Can you work these out from the drawing? Everything is in mm from the part's minimum corner. A direction names the side the tool comes from. Round coordinates to 2 decimals unless told otherwise and drop trailing zeros. Loops run counter-clockwise (first coordinate to the right, second up) from the corner with the lowest first, then second, coordinate; pieces in that order, holes last. Notation, with made-up numbers: (55.5, 17.25) -> (64.5, 17.25) arc R6 cw to (64.5, 21.25) -> close; hole circle Ø7 at (21.5, 47). An arc over 180 degrees is marked (long way). One line per item, written item: value.
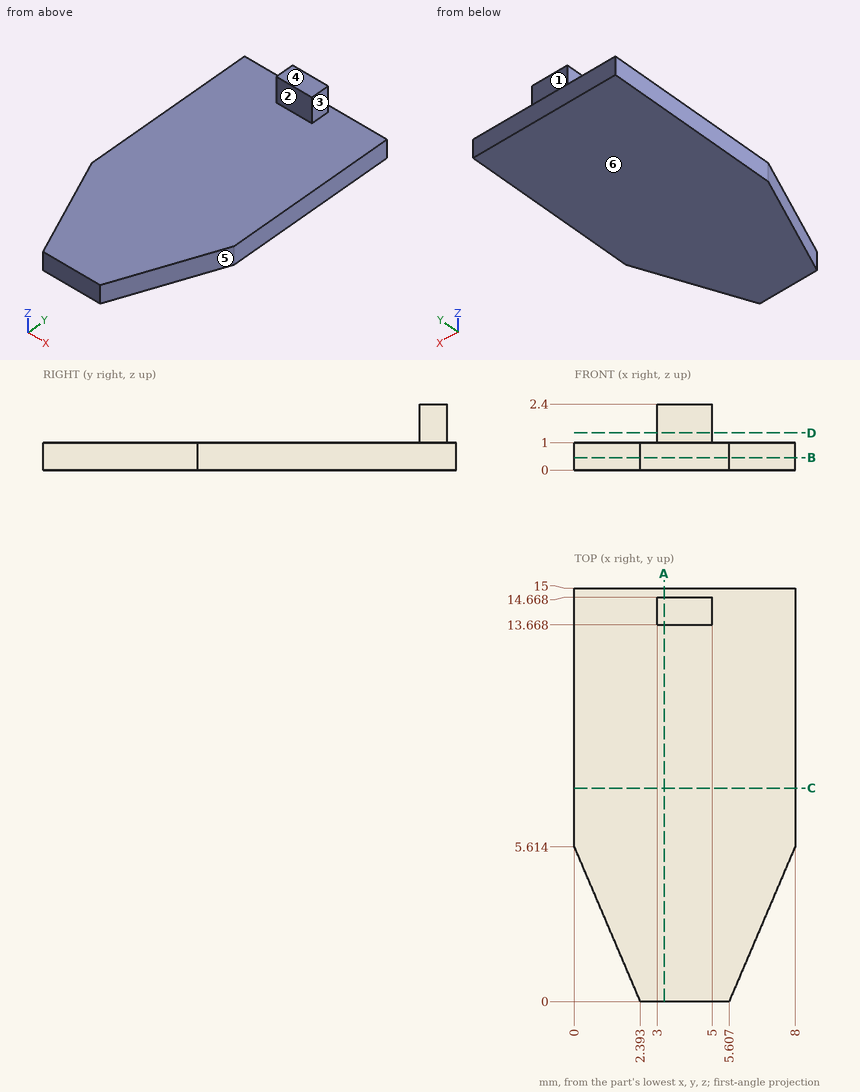
Item 1: If we section it at B-B on z = 0.45: List the corners of the cut face in (x, y) for me, plus the area to 3 significant figures.
Output:
outline: (0, 5.61) -> (2.39, 0) -> (5.61, 0) -> (8, 5.61) -> (8, 15) -> (0, 15) -> close
area: 107 mm²
Item 2: For the marked faces 1, 2 and 3, which set-ups out of +Z, -Z, +X, -X, +Y, -Y let a thin tool reach every point of the face, with its end or its side?
Output:
face 1: +Z, +X, -X, +Y
face 2: +Z, +X, -X, -Y
face 3: +Z, +X, +Y, -Y
Item 3: If we section it at C-C on y = 7.75: List the corners of the cut face in (x, z) for me.
Output:
outline: (0, 0) -> (8, 0) -> (8, 1) -> (0, 1) -> close
Item 4: Will these pins go through, and if not, where does the flat tip stop? pin 1 Ø1.1 at (x, z) = (4, 1.5) entering from +Y; pin 2 Ø1 at (x, y) = (1, 3) entering from +Z; pin 3 Ø0.7 at (x, z) = (4, 1.5) entering from -Y.
Output:
pin 1: stops at y = 15
pin 2: stops at z = 1
pin 3: stops at y = 13.67
Item 5: If we mould it in two halves opening along Z, with no side actions, what happens to the marked faces 4, 5 and 6? For each: released by +Z, released by -Z, zero draft, split by the parting line, or undercut.
Output:
face 4: released by +Z
face 5: zero draft
face 6: released by -Z
Item 6: If we section it at D-D on z = 1.35: List the corners of the cut face in (x, y) for me, plus the area to 3 significant figures.
Output:
outline: (3, 13.67) -> (5, 13.67) -> (5, 14.67) -> (3, 14.67) -> close
area: 2.00 mm²
Item 7: I need wall thicknesses on line 1 (X direction, y = 14, z = 1.25); line 2 (Z direction, x = 4, y = 3.75); line 3 (Y direction, x = 3.75, z = 1.65). Which ranges of each line are inside material? Lowest first, please. Write a range as from..to.
Output:
line 1: x = 3..5
line 2: z = 0..1
line 3: y = 13.67..14.67
Item 8: If we section it at A-A on x = 3.25: List the corners of the cut face in (y, z) for me.
Output:
outline: (0, 0) -> (15, 0) -> (15, 1) -> (14.67, 1) -> (14.67, 2.4) -> (13.67, 2.4) -> (13.67, 1) -> (0, 1) -> close
